Source: CAD feature listing. Evaluate the final solid. Frame: model axes, mm. Give positions to 0.01 mm unless a question says otherwise; leave off trailing zeros. Write each loop counter-clockwise with the first axis right and the second up, starting at its lowest first coordinate (ties: lowest second). Pieces come first, ordered by that corner, then holes. Notation, with made-up numbers: M -18,44.25 L 20,44.25 A28 cw 20,80.25 Z; hole C 48,74.25 d4. An arc over 180 degrees is marked long. Answer as a JSON object with one key per item and string values. Group by question number.
```python
from build123d import *

# Parameters (mm, degrees)
F0_R     = 71.5
F0_R_2   = 7
F0_R_3   = 6.35
F0_R_4   = 27.305
F1_DEPTH = 25.4


with BuildPart() as f1:
    # F0 (on Top) → F1 (new body)
    with BuildSketch(Plane.XY):
        Circle(F0_R)
        with Locations((-38.890873, -38.890873)):
            Circle(F0_R_2, mode=Mode.SUBTRACT)
        with Locations((0, -47.625)):
            Circle(F0_R_3, mode=Mode.SUBTRACT)
        with Locations((38.890873, -38.890873)):
            Circle(F0_R_2, mode=Mode.SUBTRACT)
        with Locations((-47.625, 0)):
            Circle(F0_R_3, mode=Mode.SUBTRACT)
        with Locations((-38.890873, 38.890873)):
            Circle(F0_R_2, mode=Mode.SUBTRACT)
        Circle(F0_R_4, mode=Mode.SUBTRACT)
        with Locations((47.625, 0)):
            Circle(F0_R_3, mode=Mode.SUBTRACT)
        with Locations((0, 47.625)):
            Circle(F0_R_3, mode=Mode.SUBTRACT)
        with Locations((38.890873, 38.890873)):
            Circle(F0_R_2, mode=Mode.SUBTRACT)
    extrude(amount=F1_DEPTH)


solid = f1.part
```
(1) Section D-D, the plane y = -25.5. Return loops of the section in (x, z), plus the area to 3 significant figures.
(2) Section A-A, the plane y = 0. Return loops of the section in (x, z) (3 decimals).
(3) Contact query for flat-ended pins moving along their axis: pin 1 Ø5 at (y, z) = (23.5, 15.5) entering from -X; pin 2 Ø8.5 at (x, y) = (-38.89, -38.89) entering from +Z; pin 3 Ø10 at (x, z) = (-41, 21) entering from +Y; pin 4 Ø20.5 at (x, y) = (-47.625, 0) entering from +Z. Output: stop coordinate, or through.
(4) Section C-C, the plane x = 20. Return loops of the section in (y, z).
(5) Pull-direction query (X, two-part tool) for faces 1 (the cylindrical face through (-52.7, 48.32, 12.52)), 2 (the cylindrical face through (-44.05, 43.62, 12.52)), 3 (the flat face through (-1, -31, 0)); classes: pulls with the +X half, pulls with the -X half, needs draft (parallel to the pull), parting line crosses it, or undercut.
(6) Ray query, L1, parallel to Y at x = 0, z = 6.75 (3 decimals); L2, parallel to X at y = 42, z = 19.25; L3, parallel to Y at x = -41, z = 11. Return the intervals inside material, ascending. Write a range as [from, to].
Reported:
{
 "1": {"outline": "M -66.8,0 L -9.76,0 L -9.76,25.4 L -66.8,25.4 Z; M 9.76,0 L 66.8,0 L 66.8,25.4 L 9.76,25.4 Z", "area": "2,900 mm2"},
 "2": {"outline": "M -71.5,0 L -53.975,0 L -53.975,25.4 L -71.5,25.4 Z; M -41.275,0 L -27.305,0 L -27.305,25.4 L -41.275,25.4 Z; M 27.305,0 L 41.275,0 L 41.275,25.4 L 27.305,25.4 Z; M 53.975,0 L 71.5,0 L 71.5,25.4 L 53.975,25.4 Z"},
 "3": {"pin 1": "stops at x = -68.35", "pin 2": "passes through", "pin 3": "stops at y = 61.78", "pin 4": "stops at z = 25.4"},
 "4": {"outline": "M -68.65,0 L -18.59,0 L -18.59,25.4 L -68.65,25.4 Z; M 18.59,0 L 68.65,0 L 68.65,25.4 L 18.59,25.4 Z"},
 "5": {"face 1": "parting line crosses it", "face 2": "undercut", "face 3": "needs draft"},
 "6": {"L1": "y = [-71.5, -53.975], [-41.275, -27.305], [27.305, 41.275], [53.975, 71.5]", "L2": "x = [-57.86, -45.16], [-32.62, -2.95], [2.95, 32.62], [45.16, 57.86]", "L3": "y = [-58.58, -45.57], [-32.22, 32.22], [45.57, 58.58]"}
}
